The figure shows three views and two pictorial views of one solid part (mm, origin at its lowest corner). Answer the questions. A direction names the side the tool comes from. Round coordinates to 2 decimals unless told otherwise and drop trailing zeros. Loops run counter-clockwise (first coordinate to the right, second up) from the corner with the lowest first, then second, coordinate; pieces in that order, holes last. Notation, with made-up numbers: (-39.75, -28.75) -> (12.25, -28.75) arc R21 ccw to (12.25, 8.25) -> close; hole circle Ø2 at (63.5, 3). An arc over 180 degrees is marked (long way). Use a Markdown table: item, result. Add a question column.
Q1. Consider line 1 (X direction, y = 29.85, z = 15); line 2 (Z direction, x = 3, y = 29); line 3 (Z direction, x = 48.5, y = 30). Determine where each line is inside the solid, lowest interval first.
Q2. Section A-A on z = 15 is taken. Give the vertices of the cut face in (x, y).
Q3. Section B-B on x = 49.9 is taken. Give the vertices of the cut face in (y, z).
Q4. Section C-C on z = 2.25 is taken. Give the vertices of the cut face in (x, y).
Q5. Which of the six approach directions +Z, -Z, +X, -X, +Y, -Y give full straight-line access (tool end or side, diameter ignored) to the marked faces 1, 2, 3, 4 and 5?
Q6. Section D-D on z = 6 is taken. Give the vertices of the cut face in (x, y), then the cut area to 3 significant figures.
Q7. Given pin 1 Ø3.5 at (x, z) = (3, 5) entering from -Y; pin 2 Ø6 at (y, z) = (10.5, 15) entering from +X; pin 3 Ø1.9 at (x, z) = (2, 14.5) entering from -Y; pin 4 Ø3 at (y, z) = (34, 11) entering from -X, each flat-ended and moving along its own axis, determine where each tip first touches the part or whether it passes through.
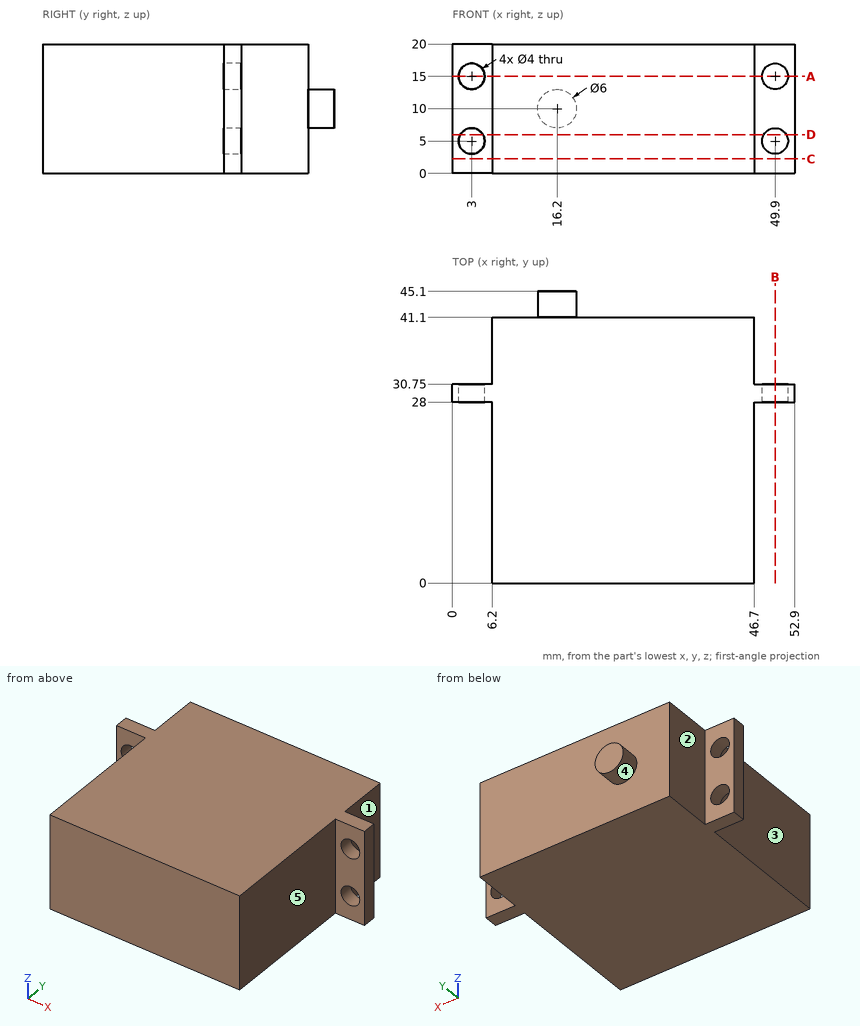
Checked values:
| question | item | result |
|---|---|---|
| 1 | line 1 | x = 0 to 1, 5 to 47.9, 51.9 to 52.9 |
| 1 | line 2 | z = 0 to 3, 7 to 13, 17 to 20 |
| 1 | line 3 | z = 0 to 3.57, 6.43 to 13.57, 16.43 to 20 |
| 2 | outline | (0, 28) -> (1, 28) -> (1, 30.75) -> (0, 30.75) -> close; (5, 28) -> (6.2, 28) -> (6.2, 0) -> (46.7, 0) -> (46.7, 28) -> (47.9, 28) -> (47.9, 30.75) -> (46.7, 30.75) -> (46.7, 41.1) -> (6.2, 41.1) -> (6.2, 30.75) -> (5, 30.75) -> close; (51.9, 28) -> (52.9, 28) -> (52.9, 30.75) -> (51.9, 30.75) -> close |
| 3 | outline | (28, 0) -> (30.75, 0) -> (30.75, 3) -> (28, 3) -> close; (28, 7) -> (30.75, 7) -> (30.75, 13) -> (28, 13) -> close; (28, 17) -> (30.75, 17) -> (30.75, 20) -> (28, 20) -> close |
| 4 | outline | (0, 28) -> (6.2, 28) -> (6.2, 0) -> (46.7, 0) -> (46.7, 28) -> (52.9, 28) -> (52.9, 30.75) -> (46.7, 30.75) -> (46.7, 41.1) -> (6.2, 41.1) -> (6.2, 30.75) -> (0, 30.75) -> close |
| 5 | face 1 | +Z, -Z, +X, +Y |
| 5 | face 2 | +Z, -Z, -X, +Y |
| 5 | face 3 | +Z, -Z, -X, -Y |
| 5 | face 4 | +Y |
| 5 | face 5 | +Z, -Z, +X, -Y |
| 6 | outline | (0, 28) -> (1.27, 28) -> (1.27, 30.75) -> (0, 30.75) -> close; (4.73, 28) -> (6.2, 28) -> (6.2, 0) -> (46.7, 0) -> (46.7, 28) -> (48.17, 28) -> (48.17, 30.75) -> (46.7, 30.75) -> (46.7, 41.1) -> (6.2, 41.1) -> (6.2, 30.75) -> (4.73, 30.75) -> close; (51.63, 28) -> (52.9, 28) -> (52.9, 30.75) -> (51.63, 30.75) -> close |
| 6 | area | 1,680 mm2 |
| 7 | pin 1 | passes through |
| 7 | pin 2 | stops at x = 46.7 |
| 7 | pin 3 | stops at y = 28 |
| 7 | pin 4 | stops at x = 6.2 |
